Read the model definition and answer for the solid it produces. Units are mm, in the model's axes. A direction names the side the tool comes from. Coordinates: 2 decimals unless noted, no trailing zeros. Order: outer loops, then holes, each group sorted by start corner. A loop starts at its lowest first (then second) coordinate and runs counter-clockwise, first axis right, second up. Notation, with made-up numbers: (50, 43.5) - (72, 43.5) arc R17 cw to (72, 76.5) - close; hole circle Ø11 at (-24, 17.25). An arc over 180 degrees is marked (long way). Answer as a JSON object with one key per item and string values. Group by question number.
from build123d import *

# Parameters (mm, degrees)
F1_W     = 77.5
F1_H     = 3.475
F1_R     = 21
F1_R_2   = 43
F1_R_3   = 16.5
F2_DEPTH = 6.1
F3_DEPTH = 2.5


with BuildPart() as f2:
    # F1 (on Front) → F2 (new body)
    with BuildSketch(Plane.XZ):
        Polygon((100.5, -68.9009734364), (63.25, -38.5886058211), (63.25, 97.4589511752), (96.191884306, 138.2240265636), (44.3153656491, 138.2240265636), (23, 110.6333434582), (23, -68.9009734364), align=None)
        with BuildLine():
            Line((53.35, -27.8899289966), (53.35, -44.6062402442))
            ThreePointArc((53.35, -44.6062402442), (54.8193979899, -46.2562123774), (55.35, -48.4009734364))
            ThreePointArc((55.35, -48.4009734364), (48.605238941, -52.4703714262), (48.15, -44.6062402442))
            Line((48.15, -44.6062402442), (48.15, -27.8899289966))
            Line((48.15, -27.8899289966), (48.15, -25.6509734364))
            Line((48.15, -25.6509734364), (48.15, -23.4120178762))
            Line((48.15, -23.4120178762), (48.15, -6.6957066286))
            ThreePointArc((48.15, -6.6957066286), (48.605238941, 1.1684245535), (55.35, -2.9009734364))
            ThreePointArc((55.35, -2.9009734364), (54.8193979899, -5.0457344953), (53.35, -6.6957066286))
            Line((53.35, -6.6957066286), (53.35, -23.4120178762))
            Line((53.35, -23.4120178762), (53.35, -25.6509734364))
            Line((53.35, -25.6509734364), (53.35, -27.8899289966))
        make_face(mode=Mode.SUBTRACT)
        with BuildLine():
            Line((53.35, 98.1746025085), (53.35, 79.3937597558))
            ThreePointArc((53.35, 79.3937597558), (54.8193979899, 77.7437876226), (55.35, 75.5990265636))
            ThreePointArc((55.35, 75.5990265636), (48.605238941, 71.5296285738), (48.15, 79.3937597558))
            Line((48.15, 79.3937597558), (48.15, 98.1746025085))
            Line((48.15, 98.1746025085), (48.15, 98.3490265636))
            Line((48.15, 98.3490265636), (48.15, 98.5234506187))
            Line((48.15, 98.5234506187), (48.15, 117.3042933714))
            ThreePointArc((48.15, 117.3042933714), (48.605238941, 125.1684245535), (55.35, 121.0990265636))
            ThreePointArc((55.35, 121.0990265636), (54.8193979899, 118.9542655047), (53.35, 117.3042933714))
            Line((53.35, 117.3042933714), (53.35, 98.5234506187))
            Line((53.35, 98.5234506187), (53.35, 98.3490265636))
            Line((53.35, 98.3490265636), (53.35, 98.1746025085))
        make_face(mode=Mode.SUBTRACT)
        with Locations((61.75, -70.6384734364)):
            Rectangle(F1_W, F1_H)
        Polygon((44.3153656491, 138.2240265636), (96.191884306, 138.2240265636), (99, 141.6990265636), (47, 141.6990265636), align=None)
        with BuildLine():
            Line((100.5, -123.3759734364), (100.5, -72.3759734364))
            Line((100.5, -72.3759734364), (23, -72.3759734364))
            Line((23, -72.3759734364), (-32.0207315003, -112.894106478))
            ThreePointArc((-32.0207315003, -112.894106478), (-41.3632102296, -191.0903053398), (37.2681203413, -195.4539366155))
            Line((37.2681203413, -195.4539366155), (91.979135359, -143.2767880183))
            ThreePointArc((91.979135359, -143.2767880183), (98.2801920718, -134.200107989), (100.5, -123.3759734364))
        make_face()
        with BuildLine():
            ThreePointArc((34.2832199621, -192.3240812312), (-45.2648285285, -176.8381561958), (-4.3373528695, -106.8906928462))
            Line((-4.3373528695, -106.8906928462), (70.9764840916, -100.2894836995))
            ThreePointArc((70.9764840916, -100.2894836995), (94.11751185, -113.8297009562), (88.9942349798, -140.1469326341))
            Line((88.9942349798, -140.1469326341), (34.2832199621, -192.3240812312))
        make_face(mode=Mode.SUBTRACT)
        with BuildLine():
            Line((47, 141.6990265636), (99, 141.6990265636))
            Line((99, 141.6990265636), (99, 192.6990265636))
            ThreePointArc((99, 192.6990265636), (73, 218.6990265636), (47, 192.6990265636))
            Line((47, 192.6990265636), (47, 141.6990265636))
        make_face()
        with Locations((73, 192.6990265636)):
            Circle(F1_R, mode=Mode.SUBTRACT)
        with BuildLine():
            Line((70.9764840916, -100.2894836995), (-4.3373528695, -106.8906928462))
            ThreePointArc((-4.3373528695, -106.8906928462), (-45.2648285285, -176.8381561958), (34.2832199621, -192.3240812312))
            Line((34.2832199621, -192.3240812312), (88.9942349798, -140.1469326341))
            ThreePointArc((88.9942349798, -140.1469326341), (94.11751185, -113.8297009562), (70.9764840916, -100.2894836995))
        make_face()
        with BuildLine():
            Line((-4.016471706, -110.5516572381), (71.297365255, -103.9504480915))
            ThreePointArc((71.297365255, -103.9504480915), (90.7687801974, -115.3435111553), (86.4579323455, -137.4874601399))
            Line((86.4579323455, -137.4874601399), (31.7469173277, -189.6646087371))
            ThreePointArc((31.7469173277, -189.6646087371), (-41.9160968759, -175.3243459967), (-4.016471706, -110.5516572381))
        make_face(mode=Mode.SUBTRACT)
        with BuildLine():
            ThreePointArc((86.4579323455, -137.4874601399), (90.7687801974, -115.3435111553), (71.297365255, -103.9504480915))
            Line((71.297365255, -103.9504480915), (-4.016471706, -110.5516572381))
            ThreePointArc((-4.016471706, -110.5516572381), (-41.9160968759, -175.3243459967), (31.7469173277, -189.6646087371))
            Line((31.7469173277, -189.6646087371), (86.4579323455, -137.4874601399))
        make_face()
        with Locations((0, -156.3759734364)):
            Circle(F1_R_2, mode=Mode.SUBTRACT)
        with Locations((73, -123.3759734364)):
            Circle(F1_R_3, mode=Mode.SUBTRACT)
    extrude(amount=F2_DEPTH)

    # F1 (on Front) → F3 (cut)
    with BuildSketch(Plane.XZ):
        Polygon((44.3153656491, 138.2240265636), (96.191884306, 138.2240265636), (99, 141.6990265636), (47, 141.6990265636), align=None)
        with Locations((61.75, -70.6384734364)):
            Rectangle(F1_W, F1_H)
        with BuildLine():
            Line((70.9764840916, -100.2894836995), (-4.3373528695, -106.8906928462))
            ThreePointArc((-4.3373528695, -106.8906928462), (-45.2648285285, -176.8381561958), (34.2832199621, -192.3240812312))
            Line((34.2832199621, -192.3240812312), (88.9942349798, -140.1469326341))
            ThreePointArc((88.9942349798, -140.1469326341), (94.11751185, -113.8297009562), (70.9764840916, -100.2894836995))
        make_face()
        with BuildLine():
            Line((-4.016471706, -110.5516572381), (71.297365255, -103.9504480915))
            ThreePointArc((71.297365255, -103.9504480915), (90.7687801974, -115.3435111553), (86.4579323455, -137.4874601399))
            Line((86.4579323455, -137.4874601399), (31.7469173277, -189.6646087371))
            ThreePointArc((31.7469173277, -189.6646087371), (-41.9160968759, -175.3243459967), (-4.016471706, -110.5516572381))
        make_face(mode=Mode.SUBTRACT)
    extrude(amount=F3_DEPTH, mode=Mode.SUBTRACT)


solid = f2.part
1. A cutting plane is placed at D-D on z = 65. Write down the section's boundary in (x, y).
2. Straight lines are drawn through the part: L1, parallel to Z at x = 50.75, y = -3.25; L2, parallel to X at y = -4, z = -31; L3, parallel to Z at x = 73, y = -3.75. For each, find the intervals that lie inside material, in ascending order.
3. For faces 1 (the flat face through (59.485, -1.232, -163.211)), 2 (the flat face through (46, -6.1, -11)), determine the directions among +Z, -Z, +X, -X, +Y, -Y from which every point of the face is accessible in a straight line to the end or side of a thin tool.
4. A cutting plane is placed at C-C on y = -3.75. Write down the section's boundary in (x, z), and give its area (3 significant figures).
5. A cutting plane is placed at B-B on x = 0. Write down the section's boundary in (y, z), and give its area (3 significant figures).
6. For a pull along Z with two mould halves and no side action, classify faces 3 (the flat face through (61.256, -1.232, -166.601)), 4 (the cylindrical face through (-42.15, -3.01, -190.13)), 5 (the flat face through (64.24, -3.01, -169.73)) as pulls with the +Z half, pulls with the -Z half, needs draft (parallel to the pull), parting line crosses it, or undercut.
7. Given pin 1 (8.5 mm diameter, centred on x = 50.75, z = -2.9, fed in from +Y); pin 2 (3 mm diameter, centred on x = 64, y = -2, fed in from -Z); pin 3 (1.5 mm diameter, centred on y = -1, z = 97.5, fed in from +X); pin 4 (3 mm diameter, centred on y = -2, z = 99.5, fed in from -X), each flat-ended and moving along its own axis, determine where each tip first touches the part or whether it passes through.
8. A cutting plane is placed at A-A on z = -29. Write down the section's boundary in (x, y), and give its area (3 significant figures).
Derived:
{
 "1": {"outline": "(23, -6.1) - (63.25, -6.1) - (63.25, 0) - (23, 0) - close"},
 "2": {"L1": "z = -182.6 to -53, 1.7 to 71, 125.7 to 206.15", "L2": "x = 23 to 48.15, 53.35 to 63.25", "L3": "z = -161.38 to -139.88, -106.88 to -46.52, 109.52 to 171.7, 213.7 to 218.7"},
 "3": {"face 1": "+Y", "face 2": "+Z, -Z, +X, -X, -Y"},
 "4": {"outline": "(-32.02, -112.89) arc R54 ccw (long way) to (37.27, -195.45) - (91.98, -143.28) arc R27.5 ccw to (100.5, -123.38) - (100.5, -68.9) - (63.25, -38.59) - (63.25, 97.46) - (99, 141.7) - (99, 192.7) arc R26 ccw to (47, 192.7) - (47, 141.7) - (23, 110.63) - (23, -72.38) - close; hole circle Ø86 at (0, -156.38); hole (48.15, -44.61) arc R4.6 ccw (long way) to (53.35, -44.61) - (53.35, -6.7) arc R4.6 ccw (long way) to (48.15, -6.7) - close; hole (48.15, 79.39) arc R4.6 ccw (long way) to (53.35, 79.39) - (53.35, 117.3) arc R4.6 ccw (long way) to (48.15, 117.3) - close; hole circle Ø42 at (73, 192.7); hole circle Ø33 at (73, -123.38)", "area": "20,100 mm2"},
 "5": {"outline": "(-6.1, -210.38) - (0, -210.38) - (0, -206.05) - (-2.5, -206.05) - (-2.5, -202.38) - (0, -202.38) - (0, -199.38) - (-6.1, -199.38) - close; (-6.1, -113.38) - (0, -113.38) - (0, -110.2) - (-2.5, -110.2) - (-2.5, -106.51) - (0, -106.51) - (0, -89.31) - (-6.1, -89.31) - close", "area": "195 mm2"},
 "6": {"face 3": "undercut", "face 4": "parting line crosses it", "face 5": "pulls with the -Z half"},
 "7": {"pin 1": "passes through", "pin 2": "stops at z = -171.39", "pin 3": "stops at x = 63.89", "pin 4": "stops at x = 23"},
 "8": {"outline": "(23, -6.1) - (48.15, -6.1) - (48.15, 0) - (23, 0) - close; (53.35, -6.1) - (63.25, -6.1) - (63.25, 0) - (53.35, 0) - close", "area": "214 mm2"}
}
